Geometry check sheet. Reference: drawing and pictorial views, mm from the part's lowest x, y, z. Give positions to 0.01 mm unless a question says otherwise; leave off trailing zeros. Order: outer loops, then holes, each group sorted by start corner. A loop starts at its lowest first (then second) coordinate and runs counter-clockwise, first axis right, second up.
Item 1: Sectioned sample at A-A on y = 8.25. Record the boundary of the cut face in (x, z), and give its area (3 significant figures).
Item 2: Sectioned sample at B-B on x = 124. Record the boundary of the cut face in (y, z).
Item 3: Material ranges on line 1 along Y through (x, z) = (30, 60.5); line 2 along X through (y, z) = (9.75, 17); line 3 along X through (y, z) = (13.5, 69), recorded low to high.
Item 4: Gauge pin test, flat ends, axial feed: P1, Ø8, axis at x = 54, z = 65, coming from the +Y side; P2, Ø2, axis at y = 12.5, z = 70.5, coming from the -X side; P3, Ø2, axis at y = 15, z = 70.5, coming from the +X side. Record the tip position at first contact, or that the pin passes through.
Item 5: Sectioned sample at C-C on z = 9. Record the boundary of the cut face in (x, y).
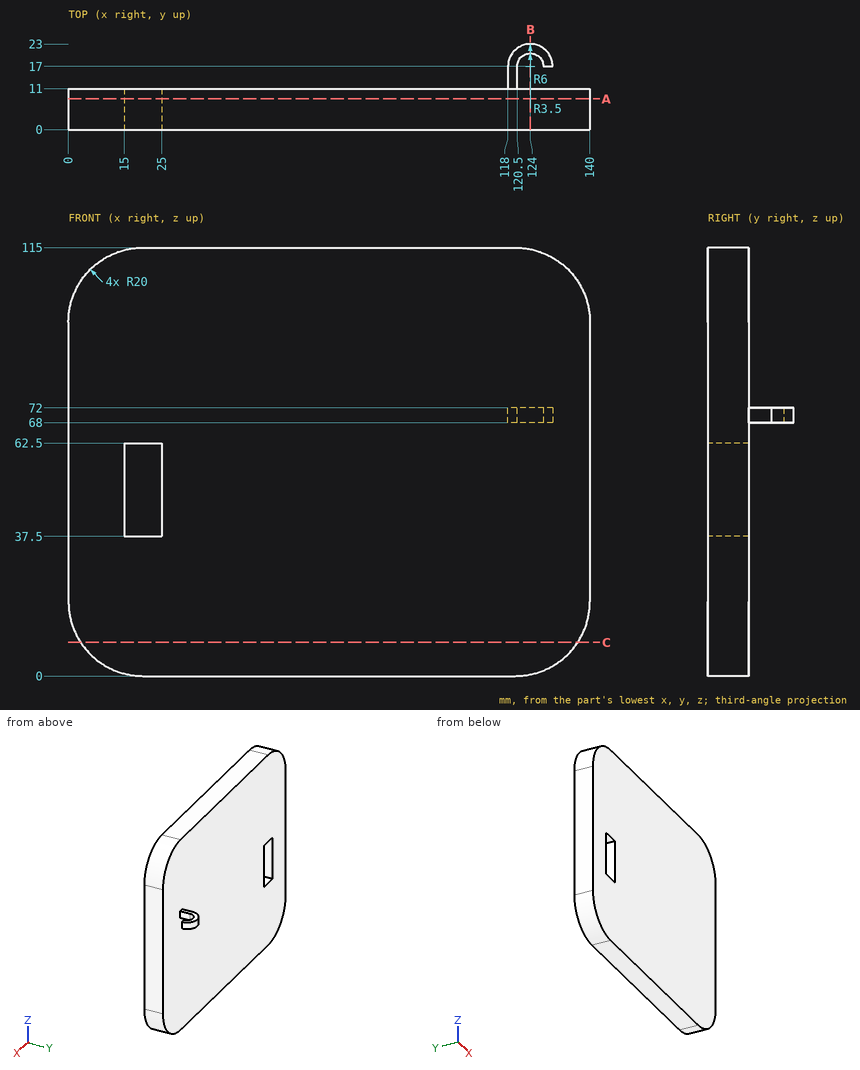
Report:
1. outline: (0, 20) arc R20 ccw to (20, 0) - (120, 0) arc R20 ccw to (140, 20) - (140, 95) arc R20 ccw to (120, 115) - (20, 115) arc R20 ccw to (0, 95) - close; hole (15, 37.5) - (25, 37.5) - (25, 62.5) - (15, 62.5) - close
1. area: 15,500 mm2
2. outline: (0, 0.4) - (11, 0.4) - (11, 114.6) - (0, 114.6) - close; (20.5, 68) - (23, 68) - (23, 72) - (20.5, 72) - close
3. line 1: y = 0 to 11
3. line 2: x = 0.23 to 139.77
3. line 3: x = 118 to 120.5
4. P1: stops at y = 11
4. P2: stops at x = 118
4. P3: stops at x = 120.5
5. outline: (3.3, 0) - (136.7, 0) - (136.7, 11) - (3.3, 11) - close
